```python
from build123d import *

# Parameters (mm, degrees)
SKETCH1_R           = 7.3
SKETCH1_R_2         = 2.1
BOSS_EXTRUDE1_DEPTH = 3
FILLET1_R           = 12
FILLET4_R           = 6
FILLET5_R           = 5
SKETCH2_R           = 1.1
CUT_EXTRUDE1_DEPTH  = 10


with BuildPart() as part:
    # Sketch1 → Boss-Extrude1 (new body)
    with BuildSketch(Plane(origin=(0, 0, 0), x_dir=(1, 0, 0), z_dir=(0, 1, 0))):
        Polygon((20, 26), (24, 22), (38, 22), (63, 19), (63, 7), (38, 4), (24, 4), (20, 0), (0, 0), (0, 26), align=None)
        with Locations((13, 13)):
            Circle(SKETCH1_R, mode=Mode.SUBTRACT)
        with Locations((38, 13)):
            Circle(SKETCH1_R_2, mode=Mode.SUBTRACT)
        with Locations((58, 13)):
            Circle(SKETCH1_R_2, mode=Mode.SUBTRACT)
    extrude(amount=BOSS_EXTRUDE1_DEPTH)

    # Fillet1
    fillet1_edges = [part.edges().sort_by_distance(p)[0] for p in [
        (0, 1.5, 0),
        (0, 1.5, -26),
    ]]
    fillet(fillet1_edges, radius=FILLET1_R)

    # Fillet4
    fillet4_edges = [part.edges().sort_by_distance(p)[0] for p in [
        (20, 1.5, -26),
        (24, 1.5, -22),
        (38, 1.5, -22),
        (38, 1.5, -4),
        (24, 1.5, -4),
        (20, 1.5, 0),
    ]]
    fillet(fillet4_edges, radius=FILLET4_R)

    # Fillet5
    fillet5_edges = [part.edges().sort_by_distance(p)[0] for p in [
        (63, 1.5, -19),
        (63, 1.5, -7),
    ]]
    fillet(fillet5_edges, radius=FILLET5_R)

    # Sketch2 → Cut-Extrude1 (cut)
    with BuildSketch(Plane(origin=(0, 3, 0), x_dir=(1, 0, 0), z_dir=(0, 1, 0))):
        with Locations((22, 13)):
            Circle(SKETCH2_R)
        with Locations((13, 4)):
            Circle(SKETCH2_R)
        with Locations((4, 13)):
            Circle(SKETCH2_R)
        with Locations((13, 22)):
            Circle(SKETCH2_R)
    extrude(amount=-CUT_EXTRUDE1_DEPTH, mode=Mode.SUBTRACT)


solid = part.part
```
Verification items for the finished model (mm, model axes). A direction names the side the tool comes from. Give positions to 0.01 mm unless a question says otherwise; leave off trailing zeros. Loops run counter-clockwise (first coordinate to the right, second up) from the corner with the lowest first, then second, coordinate; pieces in that order, holes last. Notation, with made-up numbers: M 63.25,0.25 L 83.25,0.25 A26 ccw 83.25,24.25 Z; hole C -3,64 d8. An arc over 180 degrees is marked long. Return JSON: item names as keys, results as strings.
1) Section check D-D, the plane x = 13. Enter the section's corners in (y, z), and give its area (3 significant figures).
Findings:
{"outline": "M 0,-26 L 3,-26 L 3,-23.1 L 0,-23.1 Z; M 0,-20.9 L 3,-20.9 L 3,-20.3 L 0,-20.3 Z; M 0,-5.7 L 3,-5.7 L 3,-5.1 L 0,-5.1 Z; M 0,-2.9 L 3,-2.9 L 3,0 L 0,0 Z", "area": "21.0 mm2"}
2) Section check A-A, the plane x = 58. Enter the section's corners in (y, z), and give its area (3 significant figures).
Findings:
{"outline": "M 0,-19.6 L 3,-19.6 L 3,-15.1 L 0,-15.1 Z; M 0,-10.9 L 3,-10.9 L 3,-6.4 L 0,-6.4 Z", "area": "27.0 mm2"}
3) Section check C-C, the plane y = 0.75. Enter the section's corners in (x, z).
Findings:
{"outline": "M 0,-14 A12 ccw 12,-26 L 17.51,-26 A6 ccw 21.76,-24.24 L 22.24,-23.76 A6 cw 26.49,-22 L 37.64,-22 A6 ccw 38.36,-21.96 L 58.6,-19.53 A5 ccw 63,-14.56 L 63,-11.44 A5 ccw 58.6,-6.47 L 38.36,-4.04 A6 ccw 37.64,-4 L 26.49,-4 A6 cw 22.24,-2.24 L 21.76,-1.76 A6 ccw 17.51,0 L 12,0 A12 ccw 0,-12 Z; hole C 4,-13 d2.2; hole C 13,-13 d14.6; hole C 13,-22 d2.2; hole C 13,-4 d2.2; hole C 22,-13 d2.2; hole C 38,-13 d4.2; hole C 58,-13 d4.2"}
4) Gauge pin test, flat ends, axial feed: P1, Ø3.5, axis at x = 58, z = -13, coming from the -Y side; P2, Ø1, axis at y = 1.5, z = -10, coming from the -X side; P3, Ø0.9, axis at x = 30, y = 2, coming from the +Z side. Record the tip position at first contact, or that the pin passes through.
Findings:
{"P1": "passes through", "P2": "stops at x = 0.09", "P3": "stops at z = -4"}
5) Tool access check on faces 4 (the flat face through (63, 1, -13)), 5 (the flat face through (32, 1, -22)). Record the directions out of +Z, -Z, +X, -X, +Y, -Y that give a thin tool (end or side, any length) a straight path to the whole face; none if there is none.
Findings:
{"face 4": "+Z, -Z, +X, +Y, -Y", "face 5": "-Z, +X, +Y, -Y"}
6) Material ranges on L1, parallel to X at y = 0.95, z = -13; L2, parallel to Z at x = 12, y = 1.95; L3, parallel to Z at x = 22, y = 1.2, recorded low to high. Write a range as [from, to].
Findings:
{"L1": "x = [0, 2.9], [5.1, 5.7], [20.3, 20.9], [23.1, 35.9], [40.1, 55.9], [60.1, 63]", "L2": "z = [-26, -22.46], [-21.54, -20.23], [-5.77, -4.46], [-3.54, 0]", "L3": "z = [-24, -14.1], [-11.9, -2]"}
7) Mould release check, pull along X, two halves, no side actions. Record for faces 1 (the cylindrical face through (12.189, 1.521, -4.743)), 2 (the cylindrical face through (19.78, 1.521, -25.556)), 3 (the cylindrical face through (3.61, 1.52, -22.58)): released by +X, released by -X, zero draft, split by the parting line, or undercut.
Findings:
{"face 1": "undercut", "face 2": "released by +X", "face 3": "released by -X"}
8) Section check B-B, the plane z = -13. Enter the section's corners in (x, y).
Findings:
{"outline": "M 0,0 L 2.9,0 L 2.9,3 L 0,3 Z; M 5.1,0 L 5.7,0 L 5.7,3 L 5.1,3 Z; M 20.3,0 L 20.9,0 L 20.9,3 L 20.3,3 Z; M 23.1,0 L 35.9,0 L 35.9,3 L 23.1,3 Z; M 40.1,0 L 55.9,0 L 55.9,3 L 40.1,3 Z; M 60.1,0 L 63,0 L 63,3 L 60.1,3 Z"}
